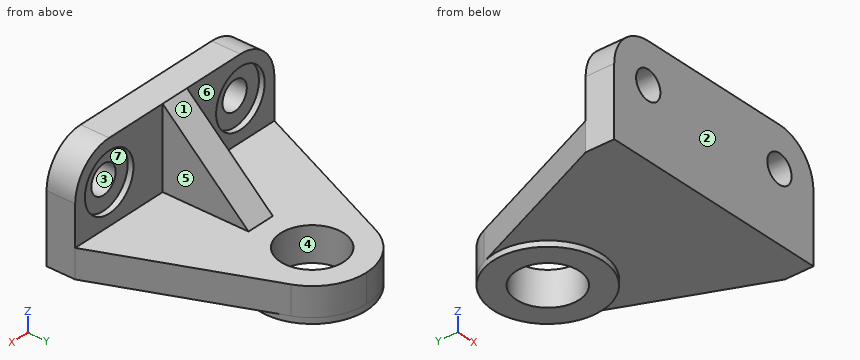
from build123d import *

# Parameters (mm, degrees)
EXTRUDE_1_DEPTH     = 41
SKETCH_2_R          = 11
CUT_EXTRUDE_1_DEPTH = 82
EXTRUDE_2_DEPTH     = 5
FILLET_1_R          = 14
CUT_EXTRUDE_2_REACH = 79
SKETCH_4_R          = 5
SKETCH_5_R          = 10
CUT_EXTRUDE_3_DEPTH = 2
SKETCH_6_R          = 19
SKETCH_6_R_2        = 11
EXTRUDE_3_DEPTH     = 2


with BuildPart() as part:
    # 스케치1 → 보스-돌출1 (new body, symmetric)
    with BuildSketch(Plane(origin=(0, 0, 0), x_dir=(0, 0, -1), z_dir=(1, 0, 0))):
        Polygon((0, 0), (38, 0), (38, 77), (28, 77), (28, 10), (0, 10), align=None)
    extrude(amount=EXTRUDE_1_DEPTH, both=True)

    # 스케치2 → 컷-돌출1 (cut)
    with BuildSketch(Plane.XY.offset(-28)):
        with BuildLine():
            Line((-41, 77), (-41, 10))
            Line((-41, 10), (-17.491366878, 65.419709208))
            ThreePointArc((-17.491366878, 65.419709208), (-10.488696893, 73.842576731), (0, 77))
            Line((0, 77), (-41, 77))
        make_face()
        with BuildLine():
            Line((41, 77), (0, 77))
            ThreePointArc((0, 77), (10.488696893, 73.842576731), (17.491366878, 65.419709208))
            Line((17.491366878, 65.419709208), (41, 10))
            Line((41, 10), (41, 77))
        make_face()
        with Locations((0, 58)):
            Circle(SKETCH_2_R)
    extrude(amount=-CUT_EXTRUDE_1_DEPTH, mode=Mode.SUBTRACT)

    # 스케치3 → 보스-돌출2 (add, symmetric)
    with BuildSketch(Plane(origin=(0, 0, 0), x_dir=(0, 0, -1), z_dir=(1, 0, 0))):
        Polygon((0, 10), (28, 10), (28, 40), align=None)
    extrude(amount=EXTRUDE_2_DEPTH, both=True)

    # 필렛1
    fillet_1_edges = [part.edges().sort_by_distance(p)[0] for p in [
        (41, 5, 0),
        (-41, 5, 0),
    ]]
    fillet(fillet_1_edges, radius=FILLET_1_R)

    # 스케치4 → 컷-돌출2 (cut, up to next)
    with BuildSketch(Plane(origin=(0, 0, 0), x_dir=(1, 0, 0), z_dir=(0, 1, 0)), mode=Mode.PRIVATE) as cut_extrude_2_sk1:
        with Locations(Location((-27, 14, 0), (0, 0, 90))):  # turned: the seam where the file's is
            Circle(SKETCH_4_R)
    cut_extrude_2_tool1 = extrude(cut_extrude_2_sk1.sketch, amount=CUT_EXTRUDE_2_REACH, mode=Mode.PRIVATE) & part.part
    add(cut_extrude_2_tool1.solids().sort_by_distance((-27, 0, -14))[0], mode=Mode.SUBTRACT)
    # 스케치4 → 컷-돌출2 (cut, up to next)
    with BuildSketch(Plane(origin=(0, 0, 0), x_dir=(1, 0, 0), z_dir=(0, 1, 0)), mode=Mode.PRIVATE) as cut_extrude_2_sk2:
        with Locations(Location((27, 14, 0), (0, 0, 90))):  # turned: the seam where the file's is
            Circle(SKETCH_4_R)
    cut_extrude_2_tool2 = extrude(cut_extrude_2_sk2.sketch, amount=CUT_EXTRUDE_2_REACH, mode=Mode.PRIVATE) & part.part
    add(cut_extrude_2_tool2.solids().sort_by_distance((27, 0, -14))[0], mode=Mode.SUBTRACT)

    # 스케치5 → 컷-돌출3 (cut)
    with BuildSketch(Plane(origin=(0, 10, 0), x_dir=(1, 0, 0), z_dir=(0, 1, 0))):
        with Locations(Location((-27, 14, 0), (0, 0, 270))):  # turned: the seam where the file's is
            Circle(SKETCH_5_R)
        with Locations(Location((27, 14, 0), (0, 0, 270))):  # turned: the seam where the file's is
            Circle(SKETCH_5_R)
    extrude(amount=-CUT_EXTRUDE_3_DEPTH, mode=Mode.SUBTRACT)

    # 스케치6 → 보스-돌출3 (add)
    with BuildSketch(Plane(origin=(0, 0, -38), x_dir=(-1, 0, 0), z_dir=(0, 0, -1))):
        with Locations(Location((0, 58, 0), (0, 0, 157.01370027))):  # turned: the seam where the file's is
            Circle(SKETCH_6_R)
        with Locations(Location((0, 58, 0), (0, 0, 180))):  # turned: the seam where the file's is
            Circle(SKETCH_6_R_2, mode=Mode.SUBTRACT)
    extrude(amount=EXTRUDE_3_DEPTH)


solid = part.part
Could you check a few things on this model? Use its own coordinates, in mm. Face numbers are marked on the shaded views. A direction names the side the tool comes from. Round coordinates to 2 decimals unless told otherwise and drop trailing zeros. Order: outer loops, then holes, each group sorted by start corner. A loop starts at its lowest first (then second) coordinate and runs counter-clockwise, first axis right, second up.
(1) I'm going to push flat-ended pins straight in: pin 1 (8.5 mm diameter, centred on y = 31.5, z = -9.5, fed in from -X); pin 2 (2 mm diameter, centred on y = 37, z = -30, fed in from +X); pin 3 (3 mm diameter, centred on y = 22, z = -19.5, fed in from +X); pin 4 (11.5 mm diameter, centred on x = 27, z = -14, fed in from +Y). Where does each tip first touch, or does it pass through?
Response values:
pin 1: passes through
pin 2: stops at x = 29.97
pin 3: stops at x = 5
pin 4: stops at y = 8
(2) Imagine slicing it at A-A (x = 23). Write out the boundary of the cut face in (y, z), plus the area to 3 significant figures.
Response values:
outline: (0, -38) - (52.43, -38) - (52.43, -28) - (10, -28) - (10, -23.17) - (8, -23.17) - (8, -17) - (0, -17) - close; (0, -11) - (8, -11) - (8, -4.83) - (10, -4.83) - (10, 0) - (0, 0) - close
area: 720 mm2
(3) If we mould it in two halves opening along Y, with no side actions, what happens to the marked faces 1, 2, 3 and 4? For each: released by +Y, released by -Y, zero draft, split by the parting line, or undercut.
Response values:
face 1: released by +Y
face 2: released by -Y
face 3: zero draft
face 4: undercut
(4) Which directions (+Z, -Z, +X, -X, +Y, -Y) give clear straight access to the entire face, cutting with the end or side of a thin tool? Please do the marked faces 5, 6 and 7.
Response values:
face 5: +Z, +X, +Y
face 6: +Z, -X, +Y
face 7: +Y
(5) Imagine slicing it at B-B (z = -33). Write out the boundary of the cut face in (x, y).
Response values:
outline: (-41, 0) - (41, 0) - (41, 10) - (17.49, 65.42) arc R19 ccw to (-17.49, 65.42) - (-41, 10) - close; hole circle Ø22 at (0, 58)
(6) Imagine slicing it at C-C (y = 58). Write out the boundary of the cut face in (x, z).
Response values:
outline: (-20.64, -38) - (-19, -38) - (-19, -40) - (-11, -40) - (-11, -28) - (-20.64, -28) - close; (11, -40) - (19, -40) - (19, -38) - (20.64, -38) - (20.64, -28) - (11, -28) - close
(7) Imagine slicing it at D-D (z = -16). Write out the boundary of the cut face in (x, y), plus the area to 3 significant figures.
Response values:
outline: (-41, 0) - (-31.58, 0) - (-31.58, 8) - (-36.8, 8) - (-36.8, 10) - (-41, 10) - close; (-22.42, 0) - (22.42, 0) - (22.42, 8) - (17.2, 8) - (17.2, 10) - (5, 10) - (5, 27.14) - (-5, 27.14) - (-5, 10) - (-17.2, 10) - (-17.2, 8) - (-22.42, 8) - close; (31.58, 0) - (41, 0) - (41, 10) - (36.8, 10) - (36.8, 8) - (31.58, 8) - close
area: 766 mm2
(8) Please list where these lines run through material, in increasing order: line 1 along Z through (x, y) = (27, 6); line 2 along Z through (x, y) = (21, 12); line 3 along Y through (x, z) = (-36.5, -22.5).
Response values:
line 1: z = -38 to -19, -9 to 0
line 2: z = -38 to -28
line 3: y = 0 to 10
